Part model, mm, in its own coordinate system. Round coordinates to 2 decimals unless told otherwise and drop trailing zeros. Order: outer loops, then holes, each group sorted by start corner. A loop starts at its lowest first (then second) coordinate and runs counter-clockwise, first axis right, second up. Notation, with made-up numbers: (83.5, 54) - (135.5, 54) arc R23 ccw to (135.5, 89) - close; hole circle Ø5 at (88.5, 15). An arc over 180 degrees is marked (long way). Return JSON: item names as keys, results as strings. Group by question number.
Item 1: Probe probe 1 along Y at (x, z) = (-25.5, 0.4); probe 2 along Y at (x, z) = (3.5, 0.55); probe 3 along X at (y, z) = (2, 1.1). List the from-to ranges inside material, lowest first.
Item 2: Saw through at A-A on x = 2.5. List the corners of the cut face in (y, z), and give its area (3 significant figures).
Item 3: Saw through at C-C on y = 13.5. List the corners of the cut face in (x, z).
Item 4: Saw through at D-D on x = -2. List the corners of the cut face in (y, z), and give its area (3 significant figures).
Item 5: Saw through at B-B on z = 1.2. List the corners of the cut face in (x, y).
Item 6: Drop a flat-ended pin along its axis: pin 1 (2.5 mm diameter, centred on x = 2.08, y = -25.34, fed in from +Z). Give the stop position or say it passes through.
```python
from build123d import *

# Parameters (mm, degrees)
BOSS_EXTRUDE1_DEPTH = 3
SKETCH2_R           = 1.6
CUT_EXTRUDE1_DEPTH  = 3
FILLET2_R           = 5


with BuildPart() as part:
    # Sketch1 → Boss-Extrude1 (new body)
    with BuildSketch(Plane.XY):
        Polygon((-27.9172032, 22.65625), (-27.9172032, -27.34375), (22.0827968, -27.34375), align=None)
    extrude(amount=BOSS_EXTRUDE1_DEPTH)

    # Sketch2 → Cut-Extrude1 (cut)
    with BuildSketch(Plane.XY.offset(3)):
        with Locations((-25.9172032, -17.34375)):
            Circle(SKETCH2_R)
        with Locations((-25.9172032, 2.65625)):
            Circle(SKETCH2_R)
        with Locations(Location((-17.9172032, -25.34375, 0), (0, 0, 180))):
            Circle(SKETCH2_R)
        with Locations(Location((2.0827968, -25.34375, 0), (0, 0, 180))):
            Circle(SKETCH2_R)
    extrude(amount=-CUT_EXTRUDE1_DEPTH, mode=Mode.SUBTRACT)

    # Fillet2
    fillet2_edges = [part.edges().sort_by_distance(p)[0] for p in [
        (22.0827968, -27.34375, 1.5),
        (-27.9172032, 22.65625, 1.5),
    ]]
    fillet(fillet2_edges, radius=FILLET2_R)


solid = part.part
```
Filled in:
{
 "1": {"probe 1": "y = -27.34 to -18.89, -15.8 to 1.11, 4.2 to 14.87", "probe 2": "y = -27.34 to -26.09, -24.6 to -8.76", "probe 3": "x = -27.92 to -27.38, -24.46 to -7.26"},
 "2": {"outline": "(-27.34, 0) - (-26.89, 0) - (-26.89, 3) - (-27.34, 3) - close; (-23.8, 0) - (-7.76, 0) - (-7.76, 3) - (-23.8, 3) - close", "area": "49.5 mm^2"},
 "3": {"outline": "(-26.98, 0) - (-18.76, 0) - (-18.76, 3) - (-26.98, 3) - close"},
 "4": {"outline": "(-27.34, 0) - (-3.26, 0) - (-3.26, 3) - (-27.34, 3) - close", "area": "72.2 mm^2"},
 "5": {"outline": "(-27.92, -27.34) - (10.01, -27.34) arc R5 ccw to (13.55, -18.81) - (-19.38, 14.12) arc R5 ccw to (-27.92, 10.59) - close; hole circle Ø3.2 at (-25.92, -17.34); hole circle Ø3.2 at (-25.92, 2.66); hole circle Ø3.2 at (-17.92, -25.34); hole circle Ø3.2 at (2.08, -25.34)"},
 "6": {"pin 1": "passes through"}
}
